```python
from build123d import *

# Parameters (mm, degrees)
SKETCH1_R               = 32.5
BOSS_EXTRUDE1_DEPTH     = 6.35
ESQUISSE1_R             = 2.54
ENL_V_MAT_EXTRU_1_DEPTH = 47.398518295
ESQUISSE3_R             = 1.75
ENL_V_MAT_EXTRU_2_DEPTH = 47.398518295


with BuildPart() as part:
    # Sketch1 → Boss-Extrude1 (new body)
    with BuildSketch(Plane(origin=(0, 0, 0), x_dir=(1, 0, 0), z_dir=(0, 1, 0))):
        with Locations(Location((0, 0, 0), (0, 0, 270))):
            Circle(SKETCH1_R)
    extrude(amount=BOSS_EXTRUDE1_DEPTH)

    # Esquisse1 → Enlèv. mat.-Extru.1 (cut, through all)
    with BuildSketch(Plane(origin=(0, 6.35, 0), x_dir=(1, 0, 0), z_dir=(0, 1, 0))):
        with Locations(Location((0, 0, 0), (0, 0, 270))):
            Circle(ESQUISSE1_R)
    extrude(amount=-ENL_V_MAT_EXTRU_1_DEPTH, mode=Mode.SUBTRACT)

    # Esquisse3 → Enlèv. mat.-Extru.2 (cut, through all)
    with BuildSketch(Plane(origin=(0, 6.35, 0), x_dir=(1, 0, 0), z_dir=(0, 1, 0))):
        with Locations(Location((0, -26.25, 0), (0, 0, 270))):
            Circle(ESQUISSE3_R)
        with Locations(Location((26.25, 0, 0), (0, 0, 270))):
            Circle(ESQUISSE3_R)
        with Locations(Location((0, 26.25, 0), (0, 0, 270))):
            Circle(ESQUISSE3_R)
        with Locations(Location((-26.25, 0, 0), (0, 0, 270))):
            Circle(ESQUISSE3_R)
    extrude(amount=-ENL_V_MAT_EXTRU_2_DEPTH, mode=Mode.SUBTRACT)


solid = part.part
```
Geometry: final body of the model. Coordinates: model frame, mm. Round coordinates to 2 decimals unless told otherwise and drop trailing zeros. Write each loop counter-clockwise with the first axis right and the second up, starting at its lowest first coordinate (ties: lowest second). Pieces come first, ordered by that corner, then holes. Notation, with made-up numbers: M 76.5,12.25 L 124.5,12.25 A14 ccw 124.5,17.25 Z; hole C 81.5,16 d3. An arc over 180 degrees is marked long. Answer in a Markdown table with one row per item. Add a question column.
(1) Ray query, L1, parallel to X at y = 4, z = 0; L2, parallel to Z at x = -0.5, y = 0.5; L3, parallel to Z at x = 1.5, y = 2. Return the intervals inside material, ascending.
(2) Contact query for flat-ended pins moving along their axis: pin 1 (6 mm diameter, centred on x = 0, z = 0, fed in from +Y); pin 2 (2 mm diameter, centred on x = -2, y = 3.5, fed in from -Z); pin 3 (2 mm diameter, centred on x = 17.5, y = 1.5, fed in from -Z). Output: stop coordinate, or through.
(3) Cut plane C-C, the plane x = -26.25. Return the cut outline in (y, z).
(4) Cut plane A-A, the plane x = 0. Return the cut outline in (y, z).
(5) Draft query along Z for faces 1 (the face through (0, 0, 7)), 2 (the face through (-24.515, 3.219, -0.228)), 3 (the face through (9.76, 3.13, 31)). Return one class per face: pulls with the +Z half, pulls with the -Z half, needs draft (parallel to the pull), parting line crosses it, or undercut.
(6) Cut plane D-D, the plane y = 5.5. Return the cut outline in (x, z), then the cut area to 3 significant figures.
(7) Cut plane B-B, the plane z = 0. Return the cut outline in (x, y).
Established:
| question | item | result |
|---|---|---|
| 1 | L1 | -32.5 to -28, -24.5 to -2.54, 2.54 to 24.5, 28 to 32.5 |
| 1 | L2 | -32.5 to -27.93, -24.57 to -2.49, 2.49 to 24.57, 27.93 to 32.5 |
| 1 | L3 | -32.47 to -27.15, -25.35 to -2.05, 2.05 to 25.35, 27.15 to 32.47 |
| 2 | pin 1 | y = 6.35 |
| 2 | pin 2 | z = -32.48 |
| 2 | pin 3 | z = -28 |
| 3 | outline | M 0,-19.16 L 6.35,-19.16 L 6.35,-1.75 L 0,-1.75 Z; M 0,1.75 L 6.35,1.75 L 6.35,19.16 L 0,19.16 Z |
| 4 | outline | M 0,-32.5 L 6.35,-32.5 L 6.35,-28 L 0,-28 Z; M 0,-24.5 L 6.35,-24.5 L 6.35,-2.54 L 0,-2.54 Z; M 0,2.54 L 6.35,2.54 L 6.35,24.5 L 0,24.5 Z; M 0,28 L 6.35,28 L 6.35,32.5 L 0,32.5 Z |
| 5 | face 1 | needs draft |
| 5 | face 2 | undercut |
| 5 | face 3 | parting line crosses it |
| 6 | outline | C 0,0 d65; hole C -26.25,0 d3.5; hole C 0,0 d5.08; hole C 0,-26.25 d3.5; hole C 0,26.25 d3.5; hole C 26.25,0 d3.5 |
| 6 | area | 3,260 mm² |
| 7 | outline | M -32.5,0 L -28,0 L -28,6.35 L -32.5,6.35 Z; M -24.5,0 L -2.54,0 L -2.54,6.35 L -24.5,6.35 Z; M 2.54,0 L 24.5,0 L 24.5,6.35 L 2.54,6.35 Z; M 28,0 L 32.5,0 L 32.5,6.35 L 28,6.35 Z |
